Verification items for the finished model (mm, model axes). A direction names the side the tool comes from. Coordinates: 2 decimals unless noted, no trailing zeros. Loops run counter-clockwise (first coordinate to the right, second up) from the corner with the lowest first, then second, coordinate; pieces in that order, holes last. Notation, with made-up numbers: (-4.75, 53) -> (38.25, 53) arc R13 ccw to (38.25, 62) -> close; hole circle Ø10 at (-28.5, 78.5). An arc over 180 degrees is marked (long way). Write item = value, one per line.
```python
from build123d import *

# Parameters (mm, degrees)
F1_DEPTH = 20
F2_R     = 2.5
F3_DEPTH = 25
F4_R     = 2


with BuildPart() as f1:
    # F0 (on Top) → F1 (new body)
    with BuildSketch(Plane.XY):
        Polygon((70, 0), (0, 0), (0, -6), (22, -6), (22, -17), (0, -17), (0, -23), (28, -23), (45, -6), (70, -6), align=None)
    extrude(amount=F1_DEPTH)

    # F2 (on Front) → F3 (cut)
    with BuildSketch(Plane.XZ):
        with BuildLine():
            Line((72, 20), (60, 20))
            ThreePointArc((60, 20), (70, 10), (60, 0))
            Line((60, 0), (72, 0))
            Line((72, 0), (72, 20))
        make_face()
        with BuildLine():
            ThreePointArc((10, 0), (0, 10), (10, 20))
            Line((10, 20), (-2, 20))
            Line((-2, 20), (-2, 0))
            Line((-2, 0), (10, 0))
        make_face()
        with BuildLine():
            Line((50, 7), (60, 7))
            ThreePointArc((60, 7), (63, 10), (60, 13))
            Line((60, 13), (50, 13))
            ThreePointArc((50, 13), (47, 10), (50, 7))
        make_face()
        with Locations((10, 10)):
            Circle(F2_R)
    extrude(amount=F3_DEPTH, mode=Mode.SUBTRACT)

    # F4
    f4_edges = [f1.edges().sort_by_distance(p)[0] for p in [
        (60, -3, 20),
        (52.5, -6, 20),
        (36.5, -14.5, 20),
        (19, -23, 20),
        (10, -20, 20),
        (16, -17, 20),
        (22, -11.5, 20),
        (16, -6, 20),
        (10, -3, 20),
        (35, 0, 20),
        (36.5, -14.5, 0),
        (45, -6, 10),
        (28, -23, 10),
        (22, -11.5, 0),
    ]]
    fillet(f4_edges, radius=F4_R)


solid = f1.part
```
1) Material ranges on line 1 (Y direction, x = 14, z = 12.5); line 2 (Z direction, x = 10, y = -20.8); line 3 (Y direction, x = 63.5, z = 12), recorded low to high.
Ans:
line_1 = -23 to -17, -6 to 0
line_2 = 0 to 7.5, 12.5 to 20
line_3 = -6 to 0
2) Sectioned sample at A-A, the plane x = 54.5. Record the cut outline in (y, z).
Ans:
outline = (-6, 2) arc R2 ccw to (-4, 0) -> (-2, 0) arc R2 ccw to (0, 2) -> (0, 7) -> (-6, 7) -> close; (-6, 13) -> (0, 13) -> (0, 18) arc R2 ccw to (-2, 20) -> (-4, 20) arc R2 ccw to (-6, 18) -> close
3) Depth check by flat-ended pin: pin 1 Ø6 at (y, z) = (-14.5, 3.5) entering from -X; pin 2 Ø2 at (y, z) = (-3.5, 5.5) entering from -X; pin 3 Ø1.5 at (x, z) = (31.5, 5.5) entering from -Y; pin 4 Ø4 at (x, z) = (10, 10) entering from -Y. Enter the tip coordinate at first touch or a pass-through.
Ans:
pin_1 = 2.75
pin_2 = 0.63
pin_3 = -20.25
pin_4 = through
4) Sectioned sample at B-B, the plane z = 10. Count the separate pieces of the cut face and the enclosed holes in it, plus the area to 3 significant figures.
Ans:
separate_pieces = 4
enclosed_holes = 0
area = 637 mm2
5) Tool access check on faces 4 (the face through (55, -3, 7)), 5 (the face through (53.01, -5.43, 19.4)), 6 (the face through (56.8, -6, 13.4)), 7 (the face through (16.9, -17.57, 19.4)), 8 (the face through (14, -6, 10)). Record the directions out of +Z, -Z, +X, -X, +Y, -Y that give a thin tool (end or side, any length) a straight path to the whole face; none if there is none.
Ans:
face_4 = +Y, -Y
face_5 = +Z, +X, -Y
face_6 = +Z, -Z, +X, -Y
face_7 = +Z, -X
face_8 = +Z, -Z, -X
6) Release check for a two-part mould opening along Z. For faces 1 (the face through (0, -20, 10)), 2 (the face through (22, -11, 10)), 3 (the face through (47, -3, 10)) record: pulls with the +Z half, pulls with the -Z half, needs draft (parallel to the pull), parting line crosses it, or undercut.
Ans:
face_1 = parting line crosses it
face_2 = needs draft
face_3 = undercut
